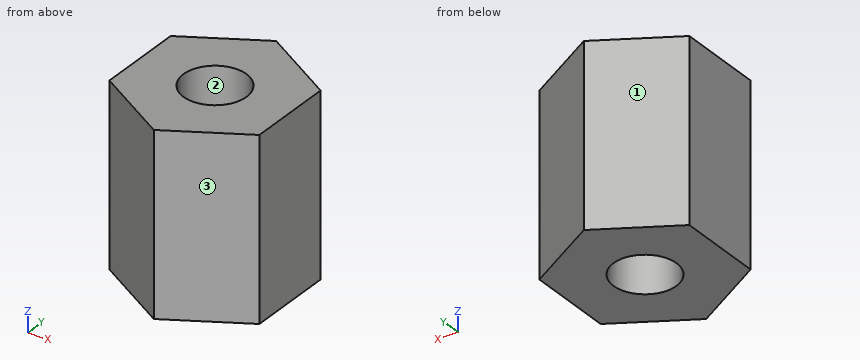
```python
from build123d import *

# Parameters (mm, degrees)
HEX_5_START      = 12.7
HEX_5_DEPTH      = 6
ROSCA_M2_5_START = 12.7
CROQUIS2_R       = 1.05
ROSCA_M2_5_DEPTH = 6


with BuildPart() as part:
    # Croquis1 → Hex_5 (new body)
    with BuildSketch(Plane.XY.offset(HEX_5_START)):
        Polygon((-105.999784659, -54.5565), (-108.5, -53.113), (-111.000215341, -54.5565), (-111.000215341, -57.4435), (-108.5, -58.887), (-105.999784659, -57.4435), align=None)
    extrude(amount=HEX_5_DEPTH)

    # Croquis2 → Rosca_M2-5 (cut)
    with BuildSketch(Plane.XY.offset(ROSCA_M2_5_START)):
        with Locations((-108.5, -56)):
            Circle(CROQUIS2_R)
    extrude(amount=ROSCA_M2_5_DEPTH, mode=Mode.SUBTRACT)


solid = part.part
```
Input: part model. Units: mm. Frame: model coordinates. Face numbers are marked on the shaded views. Coordinates: 2 decimals unless noted, no trailing zeros. Loops run counter-clockwise (first coordinate to the right, second up) from the corner with the lowest first, then second, coordinate; pieces in that order, holes last. Notation, with made-up numbers: M -3.75,13.25 L 44.25,13.25 A24 ccw 44.25,24.25 Z; hole C 66,-33 d4. An arc over 180 degrees is marked long. Use a Markdown table: item, result. Add a question column.
1) Section D-D, the plane x = -109.65. Return the cut outline in (y, z), plus the area to 3 significant figures.
2) Section A-A, the plane z = 17.85. Return the cut outline in (x, y), plus the area to 3 significant figures.
3) Line query: L1, parallel to X at y = -55.35, z = 14.6; L2, parallel to Y at x = -109.25, z = 18.55; L3, parallel to X at y = -56.95, z = 12.9. Output: solid intervals per line, ascending. Write a range as from..to.
4) Section C-C, the plane x = -108.65. Return the cut outline in (y, z).
5) Draft query along Y for the marked faces 1, 2 and 3. Return one class per face: +Y half, -Y half, draft (parallel to the pull), parting line (faces both ways), or undercut.
6) Section B-B, the plane y = -56. Return the cut outline in (x, z), plus the area to 3 significant figures.
Answer below:
| question | item | result |
|---|---|---|
| 1 | outline | M -58.22,12.7 L -53.78,12.7 L -53.78,18.7 L -58.22,18.7 Z |
| 1 | area | 26.7 mm2 |
| 2 | outline | M -111,-57.44 L -108.5,-58.89 L -106,-57.44 L -106,-54.56 L -108.5,-53.11 L -111,-54.56 Z; hole C -108.5,-56 d2.1 |
| 2 | area | 18.2 mm2 |
| 3 | L1 | -111..-109.32, -107.68..-106 |
| 3 | L2 | -58.45..-56.73, -55.27..-53.55 |
| 3 | L3 | -111..-108.95, -108.05..-106 |
| 4 | outline | M -58.8,12.7 L -57.04,12.7 L -57.04,18.7 L -58.8,18.7 Z; M -54.96,12.7 L -53.2,12.7 L -53.2,18.7 L -54.96,18.7 Z |
| 5 | face 1 | +Y half |
| 5 | face 2 | undercut |
| 5 | face 3 | -Y half |
| 6 | outline | M -111,12.7 L -109.55,12.7 L -109.55,18.7 L -111,18.7 Z; M -107.45,12.7 L -106,12.7 L -106,18.7 L -107.45,18.7 Z |
| 6 | area | 17.4 mm2 |
